Could you check a few things on this model? Use its own coordinates, in mm. A direction names the side the tool comes from. Coordinates: 2 decimals unless noted, no trailing zeros. Loops run counter-clockwise (first coordinate to the right, second up) from the corner with the lowest first, then second, coordinate; pieces in that order, holes last.
1) Imagine slicing it at B-B on y = -9.25. Please give me the cut outline in (x, z) (3 decimals).
2) Imagine slicing it at A-A on x = 125. Please give me the cut outline in (y, z).
3) For faces 1 (the face through (469.798, 0, 0)), 2 (the face through (225.41, -0.52, 3.93)), which set-ups out of +Z, -Z, +X, -X, +Y, -Y let a thin tool reach every point of the face, with its end or its side?
4) If I drill on line 1 along X through (y, z) = (-2, -4.5) (3 decimals); line 2 along Z through (x, y) = (52.5, 2); line 3 along Z through (x, y) = (6, 0), over which ranges is the centre line in solid material (lowest first)?
5) Will these pins go through, and if not, where does the flat tip stop? P1, Ø13.5, axis at y = -5.5, z = -1.5, coming from the -X side (3 decimals); P2, Ø12, axis at x = 94, y = -2, coming from the -Z side; P3, Ø2.5, axis at x = -2, y = -0.5, coming from the +Z side.
Autodesk Inventor part; units mm, degrees
ref_plane "rod_cp_XY" through (0, 0, 0) normal (1, 0, 0) x (0, 0, -1)
ref_plane "rod_cp_YZ" through (0, 0, 0) normal (0, 0, -1) x (0, 1, 0)
ref_plane "rod_cp_ZX" through (0, 0, 0) normal (0, 1, 0) x (1, 0, 0)
sketch "Sketch_1" plane through (0, 0, 0) normal (0, 0, 1) x (1, 0, 0)
  line L0 (469.7984, 0) -> (-3.175, 0)
  line L1 (-3.175, 0) -> (-3.175, 3.9624)
  line L2 (-3.175, 3.9624) -> (447.675, 3.9624)
  line L3 (447.675, 3.9624) -> (447.675, 13.5572)
  line L4 (447.675, 13.5572) -> (469.7984, 13.5572)
  line L5 (469.7984, 13.5572) -> (469.7984, 0)
  line L6 (469.7984, 0) -> (-3.175, 0)
revolve "Revolution1" add sketch "Sketch_1" angle 360 about axis through (469.7984, 0, 0) along (1, 0, 0)
sketch "Sketch_3" plane through (0, 0, 0) normal (0, 0, 1) x (1, 0, 0)
  line L0 (-3.175, 0) -> (-15.875, 0)
  line L1 (-15.875, 0) -> (-15.875, 3.3388)
  line L2 (-15.875, 3.3388) -> (-15.2451, 3.9688)
  line L3 (-15.2451, 3.9688) -> (-3.175, 3.9688)
  line L4 (-3.175, 3.9688) -> (-3.175, 0)
  line L5 (-3.175, 0) -> (-15.875, 0)
revolve "Revolution2" add sketch "Sketch_3" angle 360 about axis through (-3.175, 0, 0) along (1, 0, 0)
thread "Thread1"
sketch "Sketch_10" plane through (-3.175, 0, 0) normal (1, 0, 0) x (0, 0, -1)
  line L0 (-7.9248, 7.9248) -> (-7.9248, -7.9248)
  line L1 (-7.9248, -7.9248) -> (7.9248, -7.9248)
  line L2 (7.9248, -7.9248) -> (7.9248, 7.9248)
  line L3 (7.9248, 7.9248) -> (-7.9248, 7.9248)
  line L4 (-3.175, 3.9624) -> (-3.175, -3.9624)
  line L5 (-3.175, -3.9624) -> (3.175, -3.9624)
  line L6 (3.175, -3.9624) -> (3.175, 3.9624)
  line L7 (3.175, 3.9624) -> (-3.175, 3.9624)
extrude "Extrusion1" cut sketch "Sketch_10" along normal blind 3.175
ref_plane "rod_cp_XY" through (0, 0, 0) normal (1, 0, 0) x (0, 0, -1)
ref_plane "rod_cp_YZ" through (0, 0, 0) normal (0, 0, -1) x (0, 1, 0)
ref_plane "rod_cp_ZX" through (0, 0, 0) normal (0, 1, 0) x (1, 0, 0)
ref_plane "to_rod_clevis_XY" through (-15.875, 0, 0) normal (1, 0, 0) x (0, 0, -1)
ref_plane "to_rod_clevis_YZ" through (-15.875, 0, 0) normal (0, 0, -1) x (0, 1, 0)
ref_plane "to_rod_clevis_ZX" through (-15.875, 0, 0) normal (0, 1, 0) x (1, 0, 0)
ref_plane "rl2_XY" through (-3.175, 0, 0) normal (1, 0, 0) x (0, 0, -1)
ref_plane "rl2_YZ" through (-3.175, 0, 0) normal (0, 0, -1) x (0, 1, 0)
ref_plane "rl2_ZX" through (-3.175, 0, 0) normal (0, 1, 0) x (1, 0, 0)
ref_plane "rl1_XY" through (-15.875, 0, 0) normal (1, 0, 0) x (0, 0, -1)
ref_plane "rl1_YZ" through (-15.875, 0, 0) normal (0, 0, -1) x (0, 1, 0)
ref_plane "rl1_ZX" through (-15.875, 0, 0) normal (0, 1, 0) x (1, 0, 0)
ref_plane "thd1_XY" through (-15.875, 3.9688, 0) normal (1, 0, 0) x (0, 0, -1)
ref_plane "thd1_YZ" through (-15.875, 3.9688, 0) normal (0, 0, -1) x (0, 1, 0)
ref_plane "thd1_ZX" through (-15.875, 3.9688, 0) normal (0, 1, 0) x (1, 0, 0)
ref_plane "thd2_XY" through (-15.875, -3.9688, 0) normal (1, 0, 0) x (0, 0, -1)
ref_plane "thd2_YZ" through (-15.875, -3.9688, 0) normal (0, 0, -1) x (0, 1, 0)
ref_plane "thd2_ZX" through (-15.875, -3.9688, 0) normal (0, 1, 0) x (1, 0, 0)
ref_plane "dia1_XY" through (-3.175, 3.9624, 0) normal (1, 0, 0) x (0, 0, -1)
ref_plane "dia1_YZ" through (-3.175, 3.9624, 0) normal (0, 0, -1) x (0, 1, 0)
ref_plane "dia1_ZX" through (-3.175, 3.9624, 0) normal (0, 1, 0) x (1, 0, 0)
ref_plane "dia2_XY" through (-3.175, -3.9624, 0) normal (1, 0, 0) x (0, 0, -1)
ref_plane "dia2_YZ" through (-3.175, -3.9624, 0) normal (0, 0, -1) x (0, 1, 0)
ref_plane "dia2_ZX" through (-3.175, -3.9624, 0) normal (0, 1, 0) x (1, 0, 0)
ref_plane "wf1_XY" through (-3.175, 0, 0) normal (1, 0, 0) x (0, 0, -1)
ref_plane "wf1_YZ" through (-3.175, 0, 0) normal (0, 0, -1) x (0, 1, 0)
ref_plane "wf1_ZX" through (-3.175, 0, 0) normal (0, 1, 0) x (1, 0, 0)
ref_plane "wf2_XY" through (0, 0, 0) normal (1, 0, 0) x (0, 0, -1)
ref_plane "wf2_YZ" through (0, 0, 0) normal (0, 0, -1) x (0, 1, 0)
ref_plane "wf2_ZX" through (0, 0, 0) normal (0, 1, 0) x (1, 0, 0)
ref_plane "hh1_XY" through (497.5606, 0, 0) normal (0, 0, 1) x (1, 0, 0)
ref_plane "hh1_YZ" through (497.5606, 0, 0) normal (1, 0, 0) x (0, 1, 0)
ref_plane "hh1_ZX" through (497.5606, 0, 0) normal (0, 1, 0) x (0, 0, 1)
ref_plane "hh2_XY" through (503.9614, 0, 0) normal (0, 0, 1) x (1, 0, 0)
ref_plane "hh2_YZ" through (503.9614, 0, 0) normal (1, 0, 0) x (0, 1, 0)
ref_plane "hh2_ZX" through (503.9614, 0, 0) normal (0, 1, 0) x (0, 0, 1)
ref_plane "dia12_XY" through (0, 0, 14.1351) normal (1, 0, 0) x (0, 0, -1)
ref_plane "dia12_YZ" through (0, 0, 14.1351) normal (0, 0, -1) x (0, 1, 0)
ref_plane "dia12_ZX" through (0, 0, 14.1351) normal (0, 1, 0) x (1, 0, 0)
ref_plane "dia22_XY" through (0, 0, -14.1351) normal (1, 0, 0) x (0, 0, -1)
ref_plane "dia22_YZ" through (0, 0, -14.1351) normal (0, 0, -1) x (0, 1, 0)
ref_plane "dia22_ZX" through (0, 0, -14.1351) normal (0, 1, 0) x (1, 0, 0)
ref_plane "wfw1_XY" through (-3.175, 0, -3.175) normal (0, 1, 0) x (1, 0, 0)
ref_plane "wfw1_YZ" through (-3.175, 0, -3.175) normal (1, 0, 0) x (0, 0, -1)
ref_plane "wfw1_ZX" through (-3.175, 0, -3.175) normal (0, 0, -1) x (0, 1, 0)
ref_plane "wfw2_XY" through (-3.175, 0, 3.175) normal (0, 1, 0) x (1, 0, 0)
ref_plane "wfw2_YZ" through (-3.175, 0, 3.175) normal (1, 0, 0) x (0, 0, -1)
ref_plane "wfw2_ZX" through (-3.175, 0, 3.175) normal (0, 0, -1) x (0, 1, 0)
properties part number "0916-DX0_rod"
Filled in:
1. outline: (447.675, -9.911) - (469.798, -9.911) - (469.798, 9.911) - (447.675, 9.911) - close
2. outline: circle Ø7.92 at (0, 0)
3. face 1: +Z, -Z, +X, +Y, -Y
3. face 2: -X
4. line 1: x = 447.675 to 469.798
4. line 2: z = -3.42 to 3.42
4. line 3: z = -3.96 to 3.96
5. P1: stops at x = -15.875
5. P2: stops at z = -3.96
5. P3: stops at z = 3.97
